```python
from build123d import *

# Parameters (mm, degrees)
BOSS_EXTRU_2_DEPTH = 2
BOSS_EXTRU_8_DEPTH = 2
BOSS_EXTRU_8_DRAFT = 1


with BuildPart() as part:
    # Esquisse1 → Boss.-Extru.2 (new body)
    with BuildSketch(Plane.XY):
        with BuildLine():
            ThreePointArc((6.427291801, -2.77307052), (5.965216185, -3.662812562), (5.380773926, -4.477418002))
            ThreePointArc((5.380773926, -4.477418002), (-5.965216185, 3.662812562), (6.427291801, -2.77307052))
        make_face()
    extrude(amount=BOSS_EXTRU_2_DEPTH)


with BuildPart() as boss_extru_8_tool:
    # Esquisse7 → Boss.-Extru.8 (with draft: the straight prism first)
    with BuildSketch(Plane(origin=(0, 0, 0), x_dir=(-1, 0, 0), z_dir=(0, 0, -1))):
        with BuildLine():
            Line((27.675381467, 39.011893522), (19.675381467, 39.011893522))
            Line((19.675381467, 39.011893522), (19.675381467, 35.011893522))
            Line((19.675381467, 35.011893522), (23.151678354, 35.011893522))
            ThreePointArc((23.151678354, 35.011893522), (19.150512425, 16.86781666), (5.736262752, 4.011893522))
            ThreePointArc((5.736262752, 4.011893522), (6.806086868, 1.636209506), (6.933004295, -0.966152912))
            ThreePointArc((6.933004295, -0.966152912), (24.093742024, 15.500152171), (27.675381467, 39.011893522))
        make_face()
    extrude(amount=-BOSS_EXTRU_8_DEPTH)
    # Boss.-Extru.8: the draft: its side faces are tilted about the plane it starts from
    boss_extru_8_sides = [boss_extru_8_tool.faces().sort_by_distance(p)[0] for p in [
        (-24.093742024, 15.500152171, 1),
        (-23.675381467, 39.011893522, 1),
        (-19.675381467, 37.011893522, 1),
        (-21.413529911, 35.011893522, 1),
        (-19.150512425, 16.86781666, 1),
        (-6.806086868, 1.636209506, 1),
    ]]
    draft(boss_extru_8_sides, Plane(origin=(0, 0, 0), x_dir=(-1, 0, 0), z_dir=(0, 0, -1)), BOSS_EXTRU_8_DRAFT)


with BuildPart() as part_1:
    add(part.part)

    # Boss.-Extru.8: add boss_extru_8_tool
    add(boss_extru_8_tool.part)


solid = part_1.part
```
Source: CAD feature listing. Evaluate the final solid. Frame: model axes, mm. Round coordinates to 2 decimals unless told otherwise and drop trailing zeros. Write each loop counter-clockwise with the first axis right and the second up, starting at its lowest first coordinate (ties: lowest second). Pieces come first, ordered by that corner, then holes. Notation, with made-up numbers: M 57,77 L 64,77 A13 ccw 64,91 Z; hole C -0.5,-9 d6. An arc over 180 degrees is marked long. Answer as a JSON object with one key per item and string values. Group by question number.
(1) First-contact query: pin 1 (1 mm diameter, centred on x = -23.5, z = 0.5, fed in from -Y). Flat tip, straight axial feed; report the tip coordinate or a pass-through.
(2) Section query C-C on y = -1.5. Output: boundary loops of the cut face in (x, z), then the cut area to 3 significant figures.
(3) Ray query, line 1 (Y direction, x = -4, z = 0.1); line 2 (Y direction, x = -7, z = 1.7); line 3 (X direction, y = 8, z = 0.65). Return the intervals inside material, ascending. Write a range as [from, to].
(4) Section query B-B on x = 3.5. Output: boundary loops of the cut face in (y, z).
(5) Section query A-A on z = 1.1. Output: boundary loops of the cut face in (x, y).
Computed values:
{
 "1": {"pin 1": "y = 13.52"},
 "2": {"outline": "M -6.84,0 L 6.84,0 L 6.84,2 L -6.84,2 Z", "area": "27.3 mm^2"},
 "3": {"line 1": "[-5.74, 5.74]", "line 2": "[-0.97, 4.72]", "line 3": "[-18.96, -11.77]"},
 "4": {"outline": "M -6.06,0 L 6.06,0 L 6.06,2 L -6.06,2 Z"},
 "5": {"outline": "M -27.69,39.03 A36.99 ccw -6.93,-0.99 A7 ccw long -5.73,4.03 A31.95 cw -23.13,34.99 L -19.66,34.99 L -19.66,39.03 Z"}
}
